Input: dimensioned drawing with shaded views. Units: mm. Origin: part minimum x, y, z. A direction names the side the tool comes from. Give positions to 0.01 mm unless a question says otherwise; leave off trailing zeros. Order: outer loops, then holes, each group sorted by start corner. A loop starts at its lowest first (then second) coordinate and runs counter-clockwise, first axis right, second up.
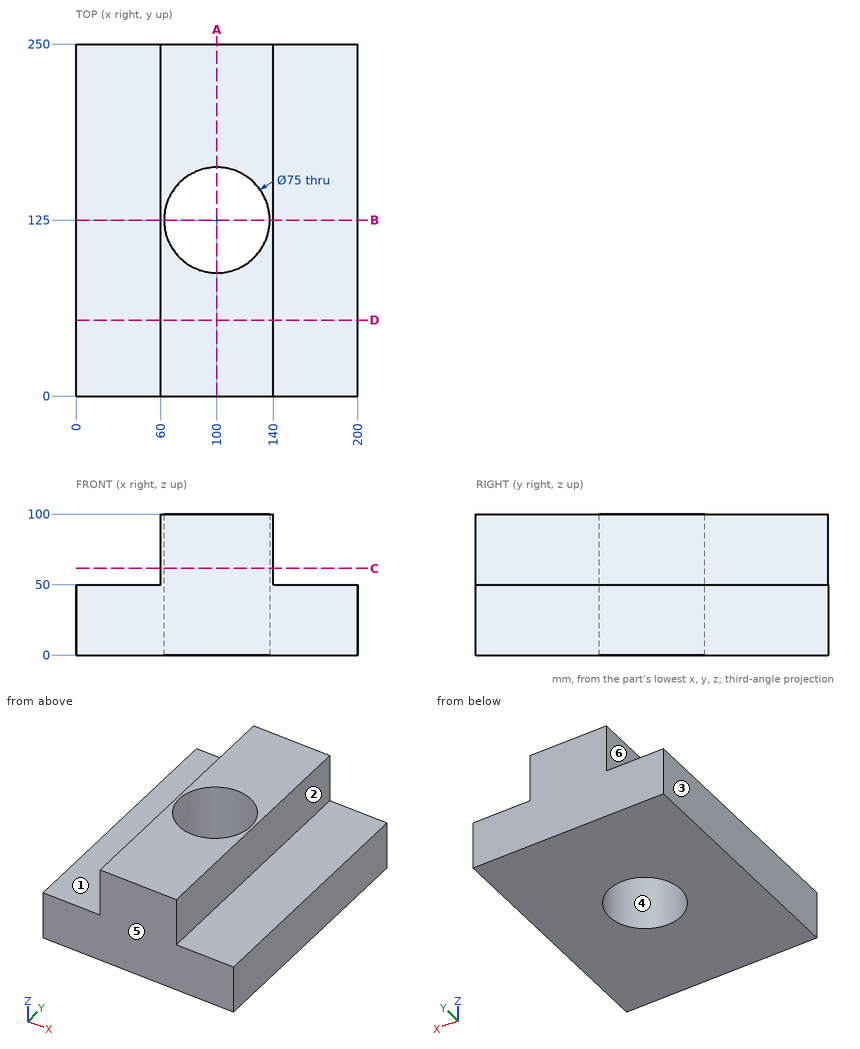
1) Cut plane B-B (y = 125). Return the cut outline in (x, z).
2) Cut plane C-C (z = 61.5). Return the cut outline in (x, y), then the cut area to 3 significant figures.
3) First-contact query: P1, Ø1.5, axis at x = 152.5, y = 132, coming from the -Z side; P2, Ø15, axis at y = 179, z = 86.5, coming from the +X side; P3, Ø15, axis at y = 186.5, z = 69.5, coming from the -X side; P4, Ø18, axis at x = 177.5, y = 70.5, coming from the +Z side. Flat tips, straight axial feed; report the tip coordinate or a pass-through.
4) Reachability of the marked faces 1, 2 and 3 from +Z, -Z, +X, -X, +Y, -Y: full face, straight path, thin tool, end or side. Return the list, or none.
5) Pull-direction query (Y, two-part tool) for the marked faces 4, 5 and 6; classes: pulls with the +Y half, pulls with the -Y half, needs draft (parallel to the pull), parting line crosses it, or undercut.
6) Line query: probe 1 along Y at (x, z) = (100, 78); probe 2 along X at (y, z) = (208.5, 71); probe 3 along Y at (x, z) = (77.5, 45). Output: solid intervals per line, ascending.
7) Cut plane D-D (y = 54). Return the cut outline in (x, z).
8) Cut plane A-A (x = 100). Return the cut outline in (y, z), then the cut area to 3 significant figures.
Geometry says:
1. outline: (0, 0) - (62.5, 0) - (62.5, 100) - (60, 100) - (60, 50) - (0, 50) - close; (137.5, 0) - (200, 0) - (200, 50) - (140, 50) - (140, 100) - (137.5, 100) - close
2. outline: (60, 0) - (140, 0) - (140, 250) - (60, 250) - close; hole circle Ø75 at (100, 125)
2. area: 15,600 mm2
3. P1: stops at z = 0
3. P2: stops at x = 140
3. P3: stops at x = 60
3. P4: stops at z = 50
4. face 1: +Z, -X, +Y, -Y
4. face 2: +Z, +X, +Y, -Y
4. face 3: +Z, -Z, -X, +Y, -Y
5. face 4: undercut
5. face 5: pulls with the -Y half
5. face 6: needs draft
6. probe 1: y = 0 to 87.5, 162.5 to 250
6. probe 2: x = 60 to 140
6. probe 3: y = 0 to 95, 155 to 250
7. outline: (0, 0) - (200, 0) - (200, 50) - (140, 50) - (140, 100) - (60, 100) - (60, 50) - (0, 50) - close
8. outline: (0, 0) - (87.5, 0) - (87.5, 100) - (0, 100) - close; (162.5, 0) - (250, 0) - (250, 100) - (162.5, 100) - close
8. area: 17,500 mm2
